```python
from build123d import *

# Parameters (mm, degrees)
SKETCH1_R           = 2.2
SKETCH1_R_2         = 1.3
BOSS_EXTRUDE1_DEPTH = 23.5
BOSS_EXTRUDE2_START = -1.5
SKETCH2_R           = 2.9
SKETCH2_R_2         = 2.2
BOSS_EXTRUDE2_DEPTH = 1.5
CUT_EXTRUDE1_START  = -3.5
CUT_EXTRUDE1_DEPTH  = 3.5
CUT_EXTRUDE2_DEPTH  = 3.5
CUT_EXTRUDE3_DEPTH  = 11.75


with BuildPart() as part:
    # Sketch1 → Boss-Extrude1 (new body)
    with BuildSketch(Plane(origin=(0, 0, 0), x_dir=(1, 0, 0), z_dir=(0, 1, 0))):
        with Locations(Location((0, 0, 0), (0, 0, 270))):
            Circle(SKETCH1_R)
        with Locations(Location((0, 0, 0), (0, 0, 270))):
            Circle(SKETCH1_R_2, mode=Mode.SUBTRACT)
    extrude(amount=BOSS_EXTRUDE1_DEPTH)

    # Sketch2 → Boss-Extrude2 (add)
    with BuildSketch(Plane(origin=(0, 16.5, 0), x_dir=(1, 0, 0), z_dir=(0, 1, 0)).offset(BOSS_EXTRUDE2_START)):
        with Locations(Location((0, 0, 0), (0, 0, 270))):
            Circle(SKETCH2_R)
        with Locations(Location((0, 0, 0), (0, 0, 270))):
            Circle(SKETCH2_R_2, mode=Mode.SUBTRACT)
    extrude(amount=BOSS_EXTRUDE2_DEPTH)

    # Sketch4 → Cut-Extrude1 (cut)
    with BuildSketch(Plane(origin=(0, 23.5, 0), x_dir=(1, 0, 0), z_dir=(0, 1, 0)).offset(CUT_EXTRUDE1_START)):
        with BuildLine():
            Line((-0.5, -1.2), (-0.5, -2.142428529))
            ThreePointArc((-0.5, -2.142428529), (0, -2.2), (0.5, -2.142428529))
            Line((0.5, -2.142428529), (0.5, -1.2))
            ThreePointArc((0.5, -1.2), (0, -1.3), (-0.5, -1.2))
        make_face()
        with BuildLine():
            ThreePointArc((0.5, 2.142428529), (0, 2.2), (-0.5, 2.142428529))
            Line((-0.5, 2.142428529), (-0.5, 1.2))
            ThreePointArc((-0.5, 1.2), (0, 1.3), (0.5, 1.2))
            Line((0.5, 1.2), (0.5, 2.142428529))
        make_face()
        with BuildLine():
            Line((-0.5, -1.2), (-0.5, -2.142428529))
            ThreePointArc((-0.5, -2.142428529), (0, -2.2), (0.5, -2.142428529))
            Line((0.5, -2.142428529), (0.5, -1.2))
            ThreePointArc((0.5, -1.2), (0, -1.3), (-0.5, -1.2))
        make_face()
        with BuildLine():
            ThreePointArc((0.5, 2.142428529), (0, 2.2), (-0.5, 2.142428529))
            Line((-0.5, 2.142428529), (-0.5, 1.2))
            ThreePointArc((-0.5, 1.2), (0, 1.3), (0.5, 1.2))
            Line((0.5, 1.2), (0.5, 2.142428529))
        make_face()
    extrude(amount=CUT_EXTRUDE1_DEPTH, mode=Mode.SUBTRACT)

    # Sketch5 → Cut-Extrude2 (cut)
    with BuildSketch(Plane.XZ):
        with BuildLine():
            ThreePointArc((0.5, 2.142428529), (0, 2.2), (-0.5, 2.142428529))
            Line((-0.5, 2.142428529), (-0.5, 1.2))
            ThreePointArc((-0.5, 1.2), (0, 1.3), (0.5, 1.2))
            Line((0.5, 1.2), (0.5, 2.142428529))
        make_face()
        with BuildLine():
            Line((-0.5, -1.2), (-0.5, -2.142428529))
            ThreePointArc((-0.5, -2.142428529), (0, -2.2), (0.5, -2.142428529))
            Line((0.5, -2.142428529), (0.5, -1.2))
            ThreePointArc((0.5, -1.2), (0, -1.3), (-0.5, -1.2))
        make_face()
        with BuildLine():
            ThreePointArc((0.5, 2.142428529), (0, 2.2), (-0.5, 2.142428529))
            Line((-0.5, 2.142428529), (-0.5, 1.2))
            ThreePointArc((-0.5, 1.2), (0, 1.3), (0.5, 1.2))
            Line((0.5, 1.2), (0.5, 2.142428529))
        make_face()
        with BuildLine():
            Line((-0.5, -1.2), (-0.5, -2.142428529))
            ThreePointArc((-0.5, -2.142428529), (0, -2.2), (0.5, -2.142428529))
            Line((0.5, -2.142428529), (0.5, -1.2))
            ThreePointArc((0.5, -1.2), (0, -1.3), (-0.5, -1.2))
        make_face()
    extrude(amount=-CUT_EXTRUDE2_DEPTH, mode=Mode.SUBTRACT)

    # Sketch6 → Cut-Extrude3 (cut, symmetric)
    with BuildSketch(Plane(origin=(0, 0, 0), x_dir=(0, 0, -1), z_dir=(1, 0, 0))):
        with BuildLine():
            Line((0.5, 10.9), (0.5, 4.9))
            ThreePointArc((0.5, 4.9), (0, 4.4), (-0.5, 4.9))
            Line((-0.5, 4.9), (-0.5, 10.9))
            ThreePointArc((-0.5, 10.9), (0, 11.4), (0.5, 10.9))
        make_face()
    extrude(amount=CUT_EXTRUDE3_DEPTH, both=True, mode=Mode.SUBTRACT)


solid = part.part
```
The model under review builds one solid part; all positions refer to its coordinate system, in mm. A direction names the side the tool comes from. Give positions to 0.01 mm unless a question says otherwise; leave off trailing zeros. Write each loop counter-clockwise with the first axis right and the second up, starting at its lowest first coordinate (ties: lowest second). Pieces come first, ordered by that corner, then holes. Notation, with made-up numbers: M 19.25,60.5 L 65.25,60.5 A14 ccw 65.25,75.5 Z; hole C 67,17 d7. An arc over 180 degrees is marked long. Answer in a Markdown table with one row per item.
Item 1: Add section D-D on z = 0.9. Give the boundary of the cut face in (x, y), plus the area to 3 significant figures.
Check sheet entries:
| item | result |
|---|---|
| outline | M -2.76,15 L -2.01,15 L -2.01,0 L -0.94,0 L -0.94,23.5 L -2.01,23.5 L -2.01,16.5 L -2.76,16.5 Z; M 0.94,0 L 2.01,0 L 2.01,15 L 2.76,15 L 2.76,16.5 L 2.01,16.5 L 2.01,23.5 L 0.94,23.5 Z |
| area | 52.5 mm2 |
Item 2: Add section B-B on y = 20.25. Give the boundary of the cut face in (x, z).
Check sheet entries:
| item | result |
|---|---|
| outline | M -0.5,-2.14 L -0.5,-1.2 A1.3 cw -0.5,1.2 L -0.5,2.14 A2.2 ccw Z; M 0.5,-2.14 A2.2 ccw 0.5,2.14 L 0.5,1.2 A1.3 cw 0.5,-1.2 Z |
Item 3: Add section A-A on z = 0. Give the boundary of the cut face in (x, y), plus the area to 3 significant figures.
Check sheet entries:
| item | result |
|---|---|
| outline | M -2.9,15 L -2.2,15 L -2.2,11.4 L -1.3,11.4 L -1.3,23.5 L -2.2,23.5 L -2.2,16.5 L -2.9,16.5 Z; M -2.2,0 L -1.3,0 L -1.3,4.4 L -2.2,4.4 Z; M 1.3,0 L 2.2,0 L 2.2,4.4 L 1.3,4.4 Z; M 1.3,11.4 L 2.2,11.4 L 2.2,15 L 2.9,15 L 2.9,16.5 L 2.2,16.5 L 2.2,23.5 L 1.3,23.5 Z |
| area | 31.8 mm2 |
Item 4: For P1, Ø3, axis at x = 0, z = -0.5, coming from the +Y side; P2, Ø2.5, axis at x = 0, z = 0, coming from the +Y side; P3, Ø0.8, axis at x = -1.5, y = 7, coming from the +Z side; P4, Ø1, axis at y = 22, z = 1.5, coming from the -X side, all flat-tipped, find the tip position at first contact; note any pin that passes through.
Check sheet entries:
| item | result |
|---|---|
| P1 | y = 23.5 |
| P2 | through |
| P3 | z = 1.91 |
| P4 | x = -1.96 |
Item 5: Tool access review of faces 1 (the face through (-1.7, 11.4, 0)), 2 (the face through (0.66, 19.95, 2.1)), 3 (the face through (0.5, 1.7, -1.7)), 4 (the face through (0.66, 7.4, 2.1)): name each direction out of +Z, -Z, +X, -X, +Y, -Y from which nothing blocks a thin tool from reaching the whole face with its end or side.
Check sheet entries:
| item | result |
|---|---|
| face 1 | +X, -X |
| face 2 | +Y |
| face 3 | +Z, -Z, -Y |
| face 4 | -Y |
Item 6: For line 1 along X through (y, z) = (17.25, 0); line 2 along Y through (x, z) = (0.3, 1.85), list the stretches that pass through material, from the lowest coordinate up.
Check sheet entries:
| item | result |
|---|---|
| line 1 | -2.2 to -1.3, 1.3 to 2.2 |
| line 2 | 3.5 to 20 |
Item 7: Add section C-C on x = 1.8. Give the boundary of the cut face in (y, z), plus the area to 3 significant figures.
Check sheet entries:
| item | result |
|---|---|
| outline | M 0,-1.26 L 15,-1.26 L 15,-2.27 L 16.5,-2.27 L 16.5,-1.26 L 23.5,-1.26 L 23.5,1.26 L 16.5,1.26 L 16.5,2.27 L 15,2.27 L 15,1.26 L 0,1.26 Z; hole M 4.9,-0.5 L 10.9,-0.5 A0.5 ccw 10.9,0.5 L 4.9,0.5 A0.5 ccw Z |
| area | 55.7 mm2 |
Item 8: Draft analysis for pull direction Y (two halves, no side actions). For faces 5 (the face through (-1.7, 4.4, 0)), 6 (the face through (2, 0, 0)), 7 (the face through (-1.7, 7.9, 0.5)), 8 (the face through (0.5, 21.7, 1.7)), state which applies: +Y half, -Y half, draft (parallel to the pull), parting line (faces both ways), or undercut.
Check sheet entries:
| item | result |
|---|---|
| face 5 | undercut |
| face 6 | -Y half |
| face 7 | undercut |
| face 8 | draft |
